Check sheet for the drawn part. Datum: minimum x, y, z corner. Units: mm. A direction names the side the tool comes from. Round coordinates to 2 decimals unless told otherwise and drop trailing zeros. Write each loop counter-clockwise with the first axis right and the second up, starting at its lowest first coordinate (ties: lowest second). Pieces come first, ordered by that corner, then holes.
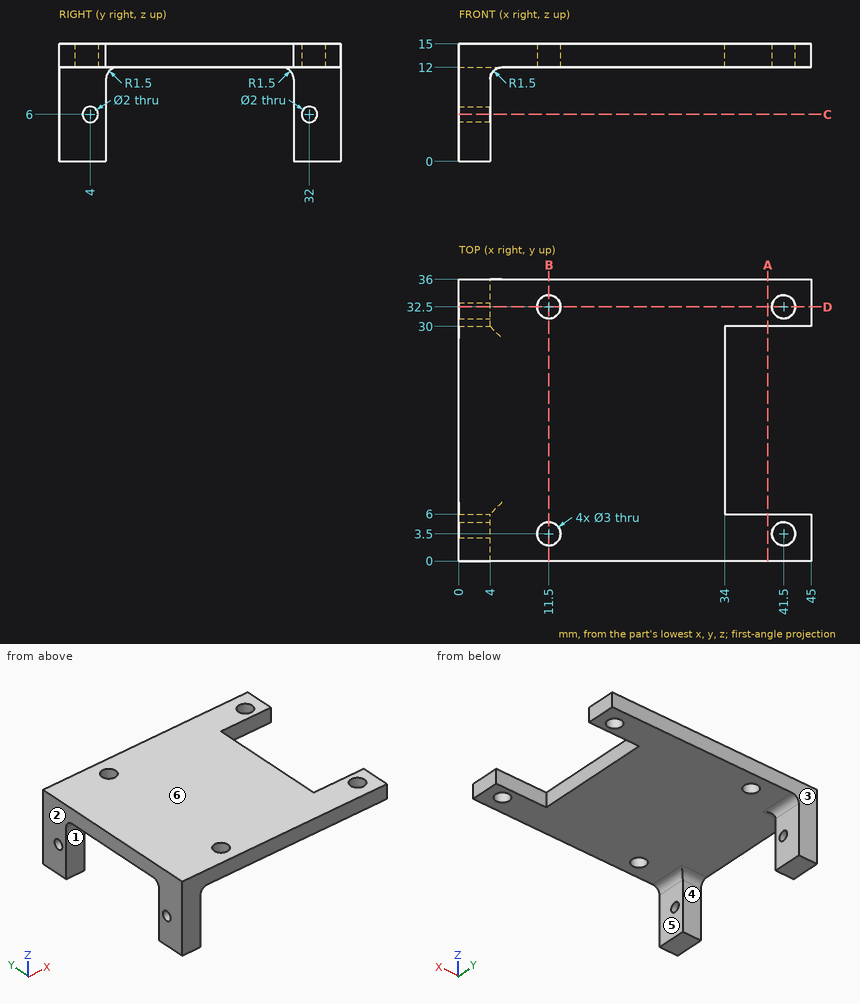
1. Sectioned sample at C-C, the plane z = 6. Enter the section's corners in (x, y), plus the area to 3 significant figures.
2. Set-up check for the marked faces 4, 5 and 6: record each of +Z, -Z, +X, -X, +Y, -Y from which the full face is reachable in a straight line by a thin tool's end or side.
3. Sectioned sample at B-B, the plane x = 11.5. Enter the section's corners in (y, z), plus the area to 3 significant figures.
4. Go/stop test with flat-tipped pins: pin 1 (18 mm diameter, centred on x = 18.5, y = 23.5, fed in from -Z); pin 2 (1.8 mm diameter, centred on x = 11.5, y = 3.5, fed in from +Z); pin 3 (1.8 mm diameter, centred on y = 4, z = 5.5, fed in from +X); pin 4 (4 mm diameter, centred on y = 24.5, z = 12, fed in from +X). Record where each tip stops, or that it passes through.
5. Release check for a two-part mould opening along Y. For the marked faces 1, 2 and 3 record: released by +Y, released by -Y, zero draft, split by the parting line, or undercut.
6. Sectioned sample at A-A, the plane x = 39.5. Enter the section's corners in (y, z).
7. Sectioned sample at D-D, the plane y = 32.5. Enter the section's corners in (x, z).
8. Scan lines: line 1 along Y through (x, z) = (41.5, 13.5); line 2 along Y through (x, z) = (11.5, 12.95); line 3 along X through (y, z) = (32.5, 13.9). Record each from-to range of solid material in increasing order.
Computed values:
1. outline: (0, 0) - (4, 0) - (4, 3) - (0, 3) - close; (0, 5) - (4, 5) - (4, 6) - (0, 6) - close; (0, 30) - (4, 30) - (4, 31) - (0, 31) - close; (0, 33) - (4, 33) - (4, 36) - (0, 36) - close
1. area: 32.0 mm2
2. face 4: -Z, +X, -X
2. face 5: -Z, +X, +Y, -Y
2. face 6: +Z, +X, -X, +Y, -Y
3. outline: (0, 12) - (2, 12) - (2, 15) - (0, 15) - close; (5, 12) - (31, 12) - (31, 15) - (5, 15) - close; (34, 12) - (36, 12) - (36, 15) - (34, 15) - close
3. area: 90.0 mm2
4. pin 1: stops at z = 12
4. pin 2: passes through
4. pin 3: stops at x = 4
4. pin 4: stops at x = 34
5. face 1: undercut
5. face 2: zero draft
5. face 3: released by +Y
6. outline: (0, 12) - (6, 12) - (6, 15) - (0, 15) - close; (30, 12) - (36, 12) - (36, 15) - (30, 15) - close
7. outline: (0, 0) - (4, 0) - (4, 5.13) - (0, 5.13) - close; (0, 6.87) - (4, 6.87) - (4, 10.5) arc R1.5 cw to (5.5, 12) - (10, 12) - (10, 15) - (0, 15) - close; (13, 12) - (40, 12) - (40, 15) - (13, 15) - close; (43, 12) - (45, 12) - (45, 15) - (43, 15) - close
8. line 1: y = 0 to 2, 5 to 6, 30 to 31, 34 to 36
8. line 2: y = 0 to 2, 5 to 31, 34 to 36
8. line 3: x = 0 to 10, 13 to 40, 43 to 45
